```python
from build123d import *

# Parameters (mm, degrees)
F0_W     = 55
F0_H     = 95
F1_DEPTH = 2
F2_W     = 4
F2_H     = 2
F3_DEPTH = 2


with BuildPart() as f1:
    # F0 (on Top) → F1 (new body)
    with BuildSketch(Plane.XY):
        Rectangle(F0_W, F0_H)
    extrude(amount=F1_DEPTH)

    # F2 (on face) → F3 (join)
    with BuildSketch(Plane.XZ.offset(47.5)):
        with Locations((17, 1)):
            Rectangle(F2_W, F2_H)
        with Locations((-17, 1)):
            Rectangle(F2_W, F2_H)
    extrude(amount=F3_DEPTH)

    # F4: F1 across plane


with BuildPart() as f1_1:
    add(f1.part)
    add(f1.part.mirror(Plane.XZ))


solid = f1_1.part
```
Source: CAD feature listing. Evaluate the final solid. Frame: model axes, mm. A direction names the side the tool comes from. Round coordinates to 2 decimals unless told otherwise and drop trailing zeros. Loops run counter-clockwise (first coordinate to the right, second up) from the corner with the lowest first, then second, coordinate; pieces in that order, holes last. Notation, with made-up numbers: (13, 22.25) - (39, 22.25) arc R11 ccw to (39, 27.25) - close; hole circle Ø11 at (71, 72.25). An arc over 180 degrees is marked (long way). Use CSV: the item, a comma, the result in double quotes.
Q1. Pin query (flat end, axial travel): pin 1 Ø1 at (x, z) = (0.5, 1) entering from -Y; pin 2 Ø1 at (x, z) = (-21.5, 1) entering from +Y; pin 3 Ø5 at (x, y) = (21.5, -15) entering from -Z; pin 4 Ø0.6 at (y, z) = (-48.5, 0.5) entering from -X. Return the tip coordinate at first contact, or that it passes through.
Reported:
pin 1,"y = -47.5"
pin 2,"y = 47.5"
pin 3,"z = 0"
pin 4,"x = -19"
Q2. Reachability of faces 1 (the flat face through (0, -47.5, 1)), 2 (the flat face through (-19, 48, 1)), 3 (the flat face through (-19, -48, 1)), 4 (the flat face through (19, -48, 1)), 5 (the flat face through (15, 48, 1)) from +Z, -Z, +X, -X, +Y, -Y: full face, straight path, thin tool, end or side. Return the list, or none.
Reported:
face 1,"+Z, -Z, -Y"
face 2,"+Z, -Z, -X, +Y"
face 3,"+Z, -Z, -X, -Y"
face 4,"+Z, -Z, +X, -Y"
face 5,"+Z, -Z, +Y"
Q3. Ray query, line 1 along Y through (x, z) = (-7, 1.6). Return the intervals inside material, ascending.
Reported:
line 1,"-47.5 to 47.5"
Q4. Section query A-A, the plane z = 1. Output: boundary loops of the cut face in (x, y), then the cut area to 3 significant figures.
Reported:
outline,"(-27.5, -47.5) - (-19, -47.5) - (-19, -49.5) - (-15, -49.5) - (-15, -47.5) - (15, -47.5) - (15, -49.5) - (19, -49.5) - (19, -47.5) - (27.5, -47.5) - (27.5, 47.5) - (19, 47.5) - (19, 49.5) - (15, 49.5) - (15, 47.5) - (-15, 47.5) - (-15, 49.5) - (-19, 49.5) - (-19, 47.5) - (-27.5, 47.5) - close"
area,"5,260 mm^2"
Q5. Section query B-B, the plane x = -5.5. Output: boundary loops of the cut face in (y, z), then the cut area to 3 significant figures.
Reported:
outline,"(-47.5, 0) - (47.5, 0) - (47.5, 2) - (-47.5, 2) - close"
area,"190 mm^2"
Q6. Mould query, pull axis X, two halves, no side actions, for faces 6 (the flat face through (15, -48, 1)), 7 (the flat face through (-17, 49.5, 1)), 8 (the flat face through (19, 48, 1)). Classes: pulls with the +X half, pulls with the -X half, needs draft (parallel to the pull), parting line crosses it, or undercut.
Reported:
face 6,"undercut"
face 7,"needs draft"
face 8,"pulls with the +X half"
